from build123d import *

# Parameters (mm, degrees)
SKETCH1_R           = 50.8
SKETCH1_R_2         = 3.175
SKETCH1_R_3         = 44.45
BOSS_EXTRUDE1_DEPTH = 6.35
SKETCH1_3_R         = 50.8
SKETCH1_3_R_2       = 44.45
CUT_EXTRUDE1_DEPTH  = 3.81
FILLET1_R           = 2.54


with BuildPart() as part:
    # Sketch1 → Boss-Extrude1 (new, symmetric)
    # profile 1 of 2: a face of its own
    with BuildSketch(Plane(origin=(0, 0, 0), x_dir=(0, 0, -1), z_dir=(1, 0, 0))):
        Circle(SKETCH1_R)
        Circle(SKETCH1_R_2, mode=Mode.SUBTRACT)
    # profile 2 of 2: a face of its own
    with BuildSketch(Plane(origin=(0, 0, 0), x_dir=(0, 0, -1), z_dir=(1, 0, 0))):
        Circle(SKETCH1_R)
        Circle(SKETCH1_R_3, mode=Mode.SUBTRACT)
    extrude(amount=BOSS_EXTRUDE1_DEPTH, both=True)

    # Sketch1<3> → Cut-Extrude1 (cut, symmetric)
    with BuildSketch(Plane(origin=(0, 0, 0), x_dir=(0, 0, -1), z_dir=(1, 0, 0))):
        Circle(SKETCH1_3_R)
        Circle(SKETCH1_3_R_2, mode=Mode.SUBTRACT)
    extrude(amount=CUT_EXTRUDE1_DEPTH, both=True, mode=Mode.SUBTRACT)

    # Fillet1
    fillet1_edges = [part.edges().sort_by_distance(p)[0] for p in [
        (-3.81, 0, 44.45),
        (3.81, 0, 44.45),
    ]]
    fillet(fillet1_edges, radius=FILLET1_R)


solid = part.part
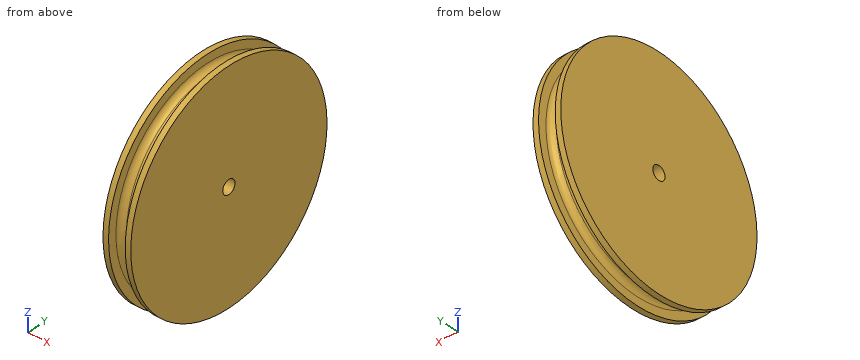
Part model, mm, in its own coordinate system. Coordinates: 2 decimals unless noted, no trailing zeros. Loops run counter-clockwise (first coordinate to the right, second up) from the corner with the lowest first, then second, coordinate; pieces in that order, holes last. Notation, with made-up numbers: M 22,57.5 L 67,57.5 A26 cw 67,75.5 Z; hole C 16,50 d3. An arc over 180 degrees is marked long. Use a Markdown table: item, result. Add a question column.
Q1. Pin check, flat tips, straight feed: P1, Ø5, axis at x = 2, z = -15, coming from the -Y side; P2, Ø2, axis at x = -1.5, z = 13, coming from the +Y side; P3, Ø1, axis at x = -3, z = 10, coming from the +Y side. Stop position of each tip, or through.
Q2. Cut at C-C (x = 5). Write the cut outline in (y, z) (3 decimals).
Q3. Cut at A-A (y = 0). Write the cut outline in (x, z) (3 decimals).
Q4. Probe L1, parallel to Y at x = -1.25, z = 0 (3 decimals); L2, parallel to Y at x = 1.5, z = 0 (3 decimals); L3, parallel to X at y = 5, z = -44.5. List the from-to ranges inside material, lowest first.
Worked out:
| question | item | result |
|---|---|---|
| 1 | P1 | stops at y = -49.03 |
| 1 | P2 | stops at y = 42.92 |
| 1 | P3 | stops at y = 44.67 |
| 2 | outline | C 0,0 d101.6; hole C 0,0 d6.35 |
| 3 | outline | M -6.35,-50.8 L -3.81,-50.8 L -3.81,-46.99 A2.54 cw -1.27,-44.45 L 1.27,-44.45 A2.54 cw 3.81,-46.99 L 3.81,-50.8 L 6.35,-50.8 L 6.35,-3.175 L -6.35,-3.175 Z; M -6.35,3.175 L 6.35,3.175 L 6.35,50.8 L 3.81,50.8 L 3.81,46.99 A2.54 cw 1.27,44.45 L -1.27,44.45 A2.54 cw -3.81,46.99 L -3.81,50.8 L -6.35,50.8 Z |
| 4 | L1 | y = -44.45 to -3.175, 3.175 to 44.45 |
| 4 | L2 | y = -44.46 to -3.175, 3.175 to 44.46 |
| 4 | L3 | x = -6.35 to -2.52, 2.52 to 6.35 |
